Here's how the part is built. I have some questions about the finished solid (model axes, mm). Face numbers are marked on the shaded views. Give positions to 0.01 mm unless a question says otherwise; leave off trailing zeros. Loops run counter-clockwise (first coordinate to the right, second up) from the corner with the lowest first, then second, coordinate; pieces in that order, holes last.
Q1. Suppose I cut it at B-B (x = 20). List the corners of the cut face in (y, z) for me, and give its area (3 significant figures).
Q2. Thinking about a two-plate mould opening in Z: for the marked faces 1, 2, 3 and 4, which applies, pulls with the +Z half, pulls with the -Z half, needs draft (parallel to the pull), parting line crosses it, or undercut?
Q3. Suppose I cut it at D-D (z = 37). List the corners of the cut face in (x, y) for me.
Q4. I need wall thicknesses on probe 1 along X at (y, z) = (137, 32.5); probe 2 along Y at (x, z) = (-20, 31); probe 3 along Z at (x, y) = (22, 137.25). Which ranges of each line are inside material? Lowest first, please.
Q5. I'm going to push flat-ended pins straight in: P1, Ø2.5, axis at x = -11.32, z = 62.31, coming from the +Y side; P2, Ø0.9, axis at x = 20.5, y = 136.5, coming from the -Z side. Where does each tip first touch, or does it pass through?
Q6. Suppose I cut it at A-A (x = 0). List the corners of the cut face in (y, z) for me.
Q7. Suppose I cut it at C-C (y = 140.25). List the corners of the cut face in (x, z) for me, and give its area (3 significant figures).
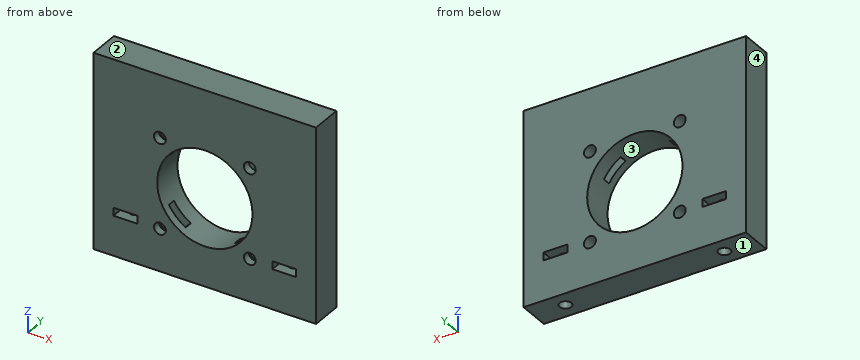
```python
from build123d import *

# Parameters (mm, degrees)
BOX775_W                     = 8
BOX775_H                     = 6
BOX775_DEPTH                 = 2
BOX776_W                     = 8
BOX776_H                     = 6
BOX776_DEPTH                 = 2
CYLINDER1869_R               = 1.5
CYLINDER1869_DEPTH           = 50
CYLINDER1869_PLACEMENT_ANGLE = 45
CYLINDER1870_R               = 1.5
CYLINDER1870_DEPTH           = 50
CYLINDER1870_PLACEMENT_ANGLE = 45
BOX770_W                     = 6
BOX770_H                     = 2
BOX770_DEPTH                 = 8
BOX766_W                     = 8
BOX766_H                     = 2
BOX766_DEPTH                 = 6
BOX768_W                     = 8
BOX768_H                     = 2
BOX768_DEPTH                 = 6
BOX769_W                     = 6
BOX769_H                     = 2
BOX769_DEPTH                 = 8
COMPOUND924_PLACEMENT_ANGLE  = 45
CYLINDER1846_R               = 12
CYLINDER1846_DEPTH           = 20
CYLINDER1848_R               = 1.5
CYLINDER1848_DEPTH           = 40
CYLINDER1850_R               = 1.5
CYLINDER1850_DEPTH           = 40
CYLINDER1849_R               = 1.5
CYLINDER1849_DEPTH           = 40
CYLINDER1847_R               = 1.5
CYLINDER1847_DEPTH           = 40
COMPOUND925_PLACEMENT_ANGLE  = 45
BOX767_W                     = 56
BOX767_H                     = 8
BOX767_DEPTH                 = 49


with BuildPart() as krychle775:
    # Box775 → Box775 (new body)
    with BuildSketch(Plane(origin=(-17, 114, 39), x_dir=(0, 1, 0), z_dir=(0, 0, 1))):
        with Locations((4, 3)):
            Rectangle(BOX775_W, BOX775_H)
    extrude(amount=BOX775_DEPTH)


with BuildPart() as compound934:
    # Box776 → Box776 (new body)
    with BuildSketch(Plane(origin=(23, 114, 39), x_dir=(0, 1, 0), z_dir=(0, 0, 1))):
        with Locations((4, 3)):
            Rectangle(BOX776_W, BOX776_H)
    extrude(amount=BOX776_DEPTH)

    # Compound934: union Krychle775
    add(krychle775.part)


with BuildPart() as compound934_1:
    # Compound934 placement: moved
    add(compound934.part.moved(Location((0, 18, 0))))


with BuildPart() as obj1:
    # Cylinder1869 → Cylinder1869 (new body)
    with BuildSketch(Plane.XY):
        Circle(CYLINDER1869_R)
    extrude(amount=CYLINDER1869_DEPTH)


with BuildPart() as obj1_1:
    # Cylinder1869 placement: moved
    add(obj1.part.moved(Location((20, 118, 0))).rotate(Axis((20, 118, 0), (0, 0, 1)), CYLINDER1869_PLACEMENT_ANGLE))


with BuildPart() as compound935:
    # Cylinder1870 → Cylinder1870 (new body)
    with BuildSketch(Plane.XY):
        Circle(CYLINDER1870_R)
    extrude(amount=CYLINDER1870_DEPTH)


with BuildPart() as compound935_1:
    # Cylinder1870 placement: moved
    add(compound935.part.moved(Location((-20, 118, 0))).rotate(Axis((-20, 118, 0), (0, 0, 1)), CYLINDER1870_PLACEMENT_ANGLE))

    # Compound935: union obj1
    add(obj1_1.part)


with BuildPart() as compound935_2:
    # Compound935 placement: moved
    add(compound935_1.part.moved(Location((0, 18, 0))))


with BuildPart() as krychle770:
    # Box770 → Box770 (new body)
    with BuildSketch(Plane(origin=(-3, 116, 30), x_dir=(1, 0, 0), z_dir=(0, 0, 1))):
        with Locations((3, 1)):
            Rectangle(BOX770_W, BOX770_H)
    extrude(amount=BOX770_DEPTH)


with BuildPart() as krychle766:
    # Box766 → Box766 (new body)
    with BuildSketch(Plane(origin=(-19, 116, 46), x_dir=(1, 0, 0), z_dir=(0, 0, 1))):
        with Locations((4, 1)):
            Rectangle(BOX766_W, BOX766_H)
    extrude(amount=BOX766_DEPTH)


with BuildPart() as krychle768:
    # Box768 → Box768 (new body)
    with BuildSketch(Plane(origin=(11, 116, 46), x_dir=(1, 0, 0), z_dir=(0, 0, 1))):
        with Locations((4, 1)):
            Rectangle(BOX768_W, BOX768_H)
    extrude(amount=BOX768_DEPTH)


with BuildPart() as compound924:
    # Box769 → Box769 (new body)
    with BuildSketch(Plane(origin=(-3, 116, 60), x_dir=(1, 0, 0), z_dir=(0, 0, 1))):
        with Locations((3, 1)):
            Rectangle(BOX769_W, BOX769_H)
    extrude(amount=BOX769_DEPTH)

    # Compound924: union Krychle770, Krychle766, Krychle768
    add(krychle770.part)
    add(krychle766.part)
    add(krychle768.part)


with BuildPart() as compound924_1:
    # Compound924 placement: moved
    add(compound924.part.moved(Location((-34.65, 0, 16.35))).rotate(Axis((-34.65, 0, 16.35), (0, 1, 0)), COMPOUND924_PLACEMENT_ANGLE))


with BuildPart() as obj2:
    # Cylinder1846 → Cylinder1846 (new body)
    with BuildSketch(Plane(origin=(0, 124, 51), x_dir=(1, 0, 0), z_dir=(0, -1, 0))):
        Circle(CYLINDER1846_R)
    extrude(amount=CYLINDER1846_DEPTH)


with BuildPart() as obj3:
    # Cylinder1848 → Cylinder1848 (new body)
    with BuildSketch(Plane(origin=(16, 140, 49), x_dir=(1, 0, 0), z_dir=(0, -1, 0))):
        Circle(CYLINDER1848_R)
    extrude(amount=CYLINDER1848_DEPTH)


with BuildPart() as obj4:
    # Cylinder1850 → Cylinder1850 (new body)
    with BuildSketch(Plane(origin=(-16, 140, 49), x_dir=(1, 0, 0), z_dir=(0, -1, 0))):
        Circle(CYLINDER1850_R)
    extrude(amount=CYLINDER1850_DEPTH)


with BuildPart() as obj5:
    # Cylinder1849 → Cylinder1849 (new body)
    with BuildSketch(Plane(origin=(0, 140, 33), x_dir=(1, 0, 0), z_dir=(0, -1, 0))):
        Circle(CYLINDER1849_R)
    extrude(amount=CYLINDER1849_DEPTH)


with BuildPart() as compound925:
    # Cylinder1847 → Cylinder1847 (new body)
    with BuildSketch(Plane(origin=(0, 140, 65), x_dir=(1, 0, 0), z_dir=(0, -1, 0))):
        Circle(CYLINDER1847_R)
    extrude(amount=CYLINDER1847_DEPTH)

    # Compound925: union obj3, obj4, obj5
    add(obj3.part)
    add(obj4.part)
    add(obj5.part)


with BuildPart() as compound925_1:
    # Compound925 placement: moved
    add(compound925.part.moved(Location((-34.65, 0, 16.35))).rotate(Axis((-34.65, 0, 16.35), (0, 1, 0)), COMPOUND925_PLACEMENT_ANGLE))


with BuildPart() as cut583:
    # Box767 → Box767 (new body)
    with BuildSketch(Plane(origin=(-28, 114, 29), x_dir=(1, 0, 0), z_dir=(0, 0, 1))):
        with Locations((28, 4)):
            Rectangle(BOX767_W, BOX767_H)
    extrude(amount=BOX767_DEPTH)

    # Cut571: cut Compound925
    add(compound925_1.part, mode=Mode.SUBTRACT)

    # Cut573: cut obj2
    add(obj2.part, mode=Mode.SUBTRACT)

    # Cut572: cut Compound924
    add(compound924_1.part, mode=Mode.SUBTRACT)


with BuildPart() as cut583_1:
    # Cut572 placement: moved
    add(cut583.part.moved(Location((0, 18, 0))))

    # Cut582: cut Compound935
    add(compound935_2.part, mode=Mode.SUBTRACT)

    # Cut583: cut Compound934
    add(compound934_1.part, mode=Mode.SUBTRACT)


with BuildPart() as cut583_2:
    # Cut583 placement: moved
    add(cut583_1.part.moved(Location((0, 1, 0))))


solid = cut583_2.part
```
Solutions:
1. outline: (133, 29) - (135.5, 29) - (135.5, 39) - (133, 39) - close; (133, 41) - (135.5, 41) - (135.5, 50) - (138.5, 50) - (138.5, 41) - (141, 41) - (141, 78) - (133, 78) - close; (138.5, 29) - (141, 29) - (141, 39) - (138.5, 39) - close
1. area: 319 mm2
2. face 1: pulls with the -Z half
2. face 2: pulls with the +Z half
2. face 3: undercut
2. face 4: needs draft
3. outline: (-28, 133) - (28, 133) - (28, 141) - (-28, 141) - close; hole circle Ø3 at (-20, 137); hole (-12.87, 135) - (-9.76, 135) - (-9.76, 137) - (-12.87, 137) - close; hole (9.75, 135) - (12.87, 135) - (12.87, 137) - (9.75, 137) - close; hole circle Ø3 at (20, 137)
4. probe 1: x = -28 to -21.5, -18.5 to 18.5, 21.5 to 28
4. probe 2: y = 133 to 135.5, 138.5 to 141
4. probe 3: z = 29 to 39, 41 to 78
5. P1: passes through
5. P2: stops at z = 50
6. outline: (133, 29) - (141, 29) - (141, 39) - (133, 39) - close; (133, 63) - (141, 63) - (141, 78) - (133, 78) - close
7. outline: (-28, 29) - (28, 29) - (28, 78) - (-28, 78) - close; hole (-23, 39) - (-17, 39) - (-17, 41) - (-23, 41) - close; hole circle Ø3 at (-11.32, 39.68); hole circle Ø3 at (-11.32, 62.31); hole circle Ø24 at (0, 51); hole circle Ø3 at (11.31, 39.68); hole circle Ø3 at (11.31, 62.31); hole (17, 39) - (23, 39) - (23, 41) - (17, 41) - close
7. area: 2,240 mm2
